Autodesk Inventor part; units mm, degrees
ref_plane "YZ Plane" through (0, 0, 0) normal (1, 0, 0) x (0, 1, 0)
ref_plane "XZ Plane" through (0, 0, 0) normal (0, 1, 0) x (-1, 0, 0)
ref_plane "XY Plane" through (0, 0, 0) normal (0, 0, 1) x (1, 0, 0)
sketch "Sketch1" plane through (0, 0, 0) normal (0, 0, 1) x (1, 0, 0)
  arc A0 (-14.9225, 0) -> (14.9225, 0) centre (0, 0) ccw
  line L0 (-14.9225, 0) -> (-14.9225, 20.6375)
  line L1 (-14.9225, 20.6375) -> (14.9225, 20.6375)
  line L2 (14.9225, 20.6375) -> (14.9225, 0)
  circle A1 centre (0, 0) radius 4.6736
  circle A2 centre (0, 0) radius 3.175
  line L3 (14.9225, 0) -> (14.9225, -0.9265)
  circle A3 centre (0, 0) radius 6.35
  dimension "d0" = 29.845
  dimension "d2" = 9.3472
  dimension "d3" = 6.35
  dimension "d6" = 12.7
  dimension "d24" = 35.56
extrude "Extrusion2" add sketch "Sketch1" against normal blind 12.7 contours L0 L1 L2 A0 | A1 | A2 | A3
extrude "Extrusion3" cut sketch "Sketch1" against normal blind 0.6096 contours A1 | A2 | A3
sketch "Sketch2" plane through (-14.9225, 20.6375, 0) normal (0, 1, 0) x (1, 0, 0)
  line L0 (0, 0) -> (0, 12.7)
  line L1 (29.845, 0) -> (0, 0)
  line L2 (29.845, 0) -> (29.845, 12.7)
  line L3 (6.0325, 10.541) -> (23.8125, 10.541)
  line L4 (23.8125, 10.541) -> (23.8125, 2.921)
  line L5 (23.8125, 2.921) -> (6.0325, 2.921)
  line L6 (6.0325, 2.921) -> (6.0325, 10.541)
  circle A0 centre (9.8425, 2.921) radius 0.381
  circle A1 centre (12.3825, 2.921) radius 0.381
  circle A2 centre (14.9225, 2.921) radius 0.381
  circle A3 centre (17.4625, 2.921) radius 0.381
  circle A4 centre (20.0025, 2.921) radius 0.381
  point P0 (14.9225, 0)
  dimension "d11" = 17.78
  dimension "d12" = 8.89
  dimension "d13" = 7.62
  dimension "d14" = 2.921
  dimension "d15" = 0.762
  dimension "d16" = 9.8425
  dimension "d19" = 2.54
  dimension "d25" = 9.8425
extrude "Extrusion4" cut sketch "Sketch2" against normal blind 1.0668 contours L3 L4 L5 A4 A3 A2 A1 A0 L6 | A0 L5 | L5 A4 | A1 L5 | L5 A3 | A2 L5 picked at (9.9376, 3.0052) picked at (19.9292, 3.1544) picked at (12.4776, 3.0052) picked at (17.3892, 3.1544) picked at (15.0176, 3.0052)
extrude "Extrusion5" add sketch "Sketch2" along normal blind 7.3152 contours A0 L5 | L5 A0 | A4 L5 | L5 A4 | A1 L5 | L5 A1 | A3 L5 | L5 A3 | A2 L5 | L5 A2
properties part number "USD S1-100-B Housing"
Could you check a few things on this model? Use its own coordinates, in mm. A direction names the side the tool comes from. Round coordinates to 2 decimals unless told otherwise and drop trailing zeros. Write each loop counter-clockwise with the first axis right and the second up, starting at its lowest first coordinate (ties: lowest second). Pieces come first, ordered by that corner, then holes. Notation, with made-up numbers: M 64.5,70.25 L 116.5,70.25 A22 ccw 116.5,81.25 Z; hole C 61.5,44.25 d10. An arc over 180 degrees is marked long. Answer in a Markdown table with one row per item. Add a question column.
Q1. Imagine slicing it at A-A (y = 23). Please give me the cut outline in (x, z), then the cut area to 3 significant figures.
Q2. If I drill on line 1 (Y direction, x = 0, z = -0.3); line 2 (X direction, y = -0.5, z = -9.75); line 3 (Z direction, x = 5.75, y = 0), over which ranges is the centre line in solid material (lowest first)? Write a range as from..to.
Q3. On a 3-axis mill with a long thin cutter (end or side, diameter ignored), from which of +Z, -Z, +X, -X, +Y, -Y can I reach the whole of each face in a straight line? I mean faces 4 (the flat face through (14.922, 10, -6)), 5 (the cylindrical face through (-1.38, -6.2, -0.3)), 6 (the flat face through (8.89, 20, -7)). Say none if no direction works.
Q4. Imagine slicing it at B-B (z = -7.5). Please give me the cut outline in (x, y) (1 decimal).
Q5. Will these pins go through, and if not, where does the flat tip stop? pin 1 Ø11.5 at (x, y) = (0, 0) entering from +Z; pin 2 Ø1.5 at (x, z) = (9.5, -2.5) entering from -Y; pin 3 Ø6.5 at (x, z) = (2, -9.5) entering from +Y; pin 4 Ø1 at (x, y) = (6.5, 15) entering from +Z.
Q6. If we mould it in two halves opening along Z, with no side actions, what happens to faces 1 (the cylindrical face through (-0.33, -14.92, -6.26)), 2 (the flat face through (-8.89, 20, -7)), 3 (the flat face through (0, 7, 0))? For each: +Z half, -Z half, draft (parallel to the pull), parting line (faces both ways), or undercut.
Q7. Imagine slicing it at D-D (y = -7.5). Please give me the cut outline in (x, z), then the cut area to 3 significant figures.
Q8. Imagine slicing it at C-C (x = -3.5). Please give me the cut outline in (y, z).
Values:
| question | item | result |
|---|---|---|
| 1 | outline | C -5.08,-2.92 d0.76; C -2.54,-2.92 d0.76; C 0,-2.92 d0.76; C 2.54,-2.92 d0.76; C 5.08,-2.92 d0.76 |
| 1 | area | 2.28 mm^2 |
| 2 | line 1 | -14.92..-6.35, 6.35..20.64 |
| 2 | line 2 | -14.91..14.91 |
| 2 | line 3 | -12.7..-0.61 |
| 3 | face 4 | +Z, -Z, +X, +Y, -Y |
| 3 | face 5 | +Z |
| 3 | face 6 | +Y |
| 4 | outline | M -14.9,0 A14.9 ccw 14.9,0 L 14.9,20.6 L 8.9,20.6 L 8.9,19.6 L -8.9,19.6 L -8.9,20.6 L -14.9,20.6 Z |
| 5 | pin 1 | z = -0.61 |
| 5 | pin 2 | y = -12.09 |
| 5 | pin 3 | y = 20.64 |
| 5 | pin 4 | z = 0 |
| 6 | face 1 | draft |
| 6 | face 2 | undercut |
| 6 | face 3 | +Z half |
| 7 | outline | M -12.9,-12.7 L 12.9,-12.7 L 12.9,0 L -12.9,0 Z |
| 7 | area | 328 mm^2 |
| 8 | outline | M -14.51,-12.7 L 20.64,-12.7 L 20.64,-10.54 L 19.57,-10.54 L 19.57,-2.92 L 20.64,-2.92 L 20.64,0 L 5.3,0 L 5.3,-0.61 L -5.3,-0.61 L -5.3,0 L -14.51,0 Z |
